Geometry check sheet. Reference: the model listing, model coordinates, mm. A direction names the side the tool comes from. Coordinates: 2 decimals unless noted, no trailing zeros. Write each loop counter-clockwise with the first axis right and the second up, starting at its lowest first coordinate (ties: lowest second). Pieces come first, ordered by that corner, then holes. Notation, with made-up numbers: (42, 42) -> (66, 42) arc R16 cw to (66, 55) -> close; hole circle Ø11 at (30.25, 85). An arc over 180 degrees is marked (long way). Answer in a Markdown table with one row per item. Add a question column.
1. Cross-section at B-B on x = 44.25. Record the cut outline in (y, z), and give its area (3 significant figures).
2. Mould release check, pull along Y, two halves, no side actions. Record for faces 1 (the flat face through (49, 18, 40.5)), 2 (the flat face through (-16, 2, -1)), 3 (the cylindrical face through (67.614, 28.25, 41.486)): pulls with the +Y half, pulls with the -Y half, needs draft (parallel to the pull), parting line crosses it, or undercut.
3. Depth check by flat-ended pin: P1, Ø17, axis at x = 40.5, y = 24, coming from the +Z side; P2, Ø1.5, axis at x = 50.5, y = 22.5, coming from the -Z side; P3, Ø3.5, axis at x = 33.25, y = 9, coming from the -Z side; P4, Ø2, axis at y = 1.5, z = 57.5, coming from the +X side. Enter the tip coordinate at first touch or a pass-through.
4. Cross-section at D-D on x = 9.25. Record the cut outline in (y, z).
5. Cross-section at A-A on z = -50. Record the cut outline in (x, y), and give its area (3 significant figures).
6. Cross-section at C-C on y = 4.5. Record the cut outline in (x, z), and give its area (3 significant figures).
7. Set-up check for faces 4 (the flat face through (48, 17, 42.5)), 5 (the cylindrical face through (67.614, 28.25, -41.514)): record each of +Z, -Z, +X, -X, +Y, -Y from which the full face is reachable in a straight line by a thin tool's end or side.
8. Scan lines: L1, parallel to Y at x = 66.25, z = 41.25; L2, parallel to X at y = 0.95, z = 71; L3, parallel to X at y = 1.6, z = -50. Record each from-to range of solid material in increasing order. Write a range as from..to.
```python
from build123d import *

# Parameters (mm, degrees)
SKETCH1_R           = 2.15
SKETCH1_R_2         = 1.75
SKETCH1_W           = 10.5
SKETCH1_H           = 6
SKETCH1_W_2         = 6
SKETCH1_H_2         = 4
SKETCH1_H_3         = 10.5
BOSS_EXTRUDE1_DEPTH = 2
SKETCH2_W           = 40
SKETCH2_H           = 2
BOSS_EXTRUDE2_DEPTH = 34
SKETCH4_R           = 1.85
SKETCH4_R_2         = 7.5
CUT_EXTRUDE2_DEPTH  = 120
SKETCH5_W           = 4.5
SKETCH5_H           = 32.5
CUT_EXTRUDE3_DEPTH  = 120


with BuildPart() as part:
    # Sketch1 → Boss-Extrude1 (new body)
    with BuildSketch(Plane(origin=(0, 0, 0), x_dir=(1, 0, 0), z_dir=(0, 1, 0))):
        Polygon((-68.75, -75), (33.25, -75), (33.25, -42.5), (68.75, -42.5), (68.75, 42.5), (33.25, 42.5), (33.25, 75), (-68.75, 75), align=None)
        with Locations(Location((-56.75, -71, 0), (0, 0, 270))):
            Circle(SKETCH1_R, mode=Mode.SUBTRACT)
        with Locations(Location((-41.97, -71, 0), (0, 0, 270))):
            Circle(SKETCH1_R, mode=Mode.SUBTRACT)
        with Locations(Location((-52.25, -40.5, 0), (0, 0, 270))):
            Circle(SKETCH1_R_2, mode=Mode.SUBTRACT)
        with Locations(Location((-29.75, -50, 0), (0, 0, 270))):
            Circle(SKETCH1_R_2, mode=Mode.SUBTRACT)
        with Locations(Location((-35.75, -19.5, 0), (0, 0, 270))):
            Circle(SKETCH1_R_2, mode=Mode.SUBTRACT)
        with Locations(Location((-26.5, -28.4, 0), (0, 0, 270))):
            Circle(SKETCH1_R_2, mode=Mode.SUBTRACT)
        with Locations(Location((-14.75, -37, 0), (0, 0, 270))):
            Circle(SKETCH1_R_2, mode=Mode.SUBTRACT)
        with Locations(Location((9.25, -50, 0), (0, 0, 270))):
            Circle(SKETCH1_R_2, mode=Mode.SUBTRACT)
        with Locations(Location((13.5, -68.4, 0), (0, 0, 270))):
            Circle(SKETCH1_R_2, mode=Mode.SUBTRACT)
        with Locations(Location((-52.25, 40.5, 0), (0, 0, 270))):
            Circle(SKETCH1_R_2, mode=Mode.SUBTRACT)
        with Locations(Location((-35.75, 19.5, 0), (0, 0, 270))):
            Circle(SKETCH1_R_2, mode=Mode.SUBTRACT)
        with Locations(Location((-56.75, 71, 0), (0, 0, 270))):
            Circle(SKETCH1_R, mode=Mode.SUBTRACT)
        with Locations(Location((-41.97, 71, 0), (0, 0, 270))):
            Circle(SKETCH1_R, mode=Mode.SUBTRACT)
        with Locations(Location((-29.75, 50, 0), (0, 0, 270))):
            Circle(SKETCH1_R_2, mode=Mode.SUBTRACT)
        with Locations(Location((-26.5, 28.4, 0), (0, 0, 270))):
            Circle(SKETCH1_R_2, mode=Mode.SUBTRACT)
        with Locations(Location((9.25, 50, 0), (0, 0, 270))):
            Circle(SKETCH1_R_2, mode=Mode.SUBTRACT)
        with Locations(Location((13.5, 68.4, 0), (0, 0, 270))):
            Circle(SKETCH1_R_2, mode=Mode.SUBTRACT)
        with Locations((-52, -61.25)):
            Rectangle(SKETCH1_W, SKETCH1_H, mode=Mode.SUBTRACT)
        with Locations((-49.92, -70)):
            Rectangle(SKETCH1_W_2, SKETCH1_H_2, mode=Mode.SUBTRACT)
        with Locations((-52, 61.25)):
            Rectangle(SKETCH1_W, SKETCH1_H, mode=Mode.SUBTRACT)
        with Locations((-49.92, 70)):
            Rectangle(SKETCH1_W_2, SKETCH1_H_2, mode=Mode.SUBTRACT)
        with Locations((61.796244223, 0)):
            Rectangle(SKETCH1_W_2, SKETCH1_H_3, mode=Mode.SUBTRACT)
    extrude(amount=BOSS_EXTRUDE1_DEPTH)

    # Sketch2 → Boss-Extrude2 (add)
    with BuildSketch(Plane(origin=(0, 0, 0), x_dir=(-1, 0, 0), z_dir=(0, -1, 0))):
        with Locations((-48.75, 41.5)):
            Rectangle(SKETCH2_W, SKETCH2_H)
        with Locations((-48.75, -41.5)):
            Rectangle(SKETCH2_W, SKETCH2_H)
    extrude(amount=-BOSS_EXTRUDE2_DEPTH)

    # Sketch4 → Cut-Extrude2 (cut)
    with BuildSketch(Plane(origin=(0, 0, -42.5), x_dir=(-1, 0, 0), z_dir=(0, 0, -1))):
        with Locations((-66.25, 27)):
            Circle(SKETCH4_R)
        with Locations((-33.25, 27)):
            Circle(SKETCH4_R)
        with Locations((-33.25, 9)):
            Circle(SKETCH4_R)
        with Locations((-66.25, 9)):
            Circle(SKETCH4_R)
        with Locations((-57.25, 18)):
            Circle(SKETCH4_R_2)
        with BuildLine():
            Line((-47, 13), (-47, 23))
            ThreePointArc((-47, 23), (-44.25, 25.75), (-41.5, 23))
            Line((-41.5, 23), (-41.5, 13))
            ThreePointArc((-41.5, 13), (-44.25, 10.25), (-47, 13))
        make_face()
    extrude(amount=-CUT_EXTRUDE2_DEPTH, mode=Mode.SUBTRACT)

    # Sketch5 → Cut-Extrude3 (cut)
    with BuildSketch(Plane(origin=(0, 2, 0), x_dir=(1, 0, 0), z_dir=(0, 1, 0))):
        with Locations((31, -58.75)):
            Rectangle(SKETCH5_W, SKETCH5_H)
        with Locations((31, 58.75)):
            Rectangle(SKETCH5_W, SKETCH5_H)
    extrude(amount=-CUT_EXTRUDE3_DEPTH, mode=Mode.SUBTRACT)


solid = part.part
```
Results found:
| question | item | result |
|---|---|---|
| 1 | outline | (0, -42.5) -> (10.25, -42.5) -> (10.25, -40.5) -> (2, -40.5) -> (2, 40.5) -> (10.25, 40.5) -> (10.25, 42.5) -> (0, 42.5) -> close; (25.75, -42.5) -> (34, -42.5) -> (34, -40.5) -> (25.75, -40.5) -> close; (25.75, 40.5) -> (34, 40.5) -> (34, 42.5) -> (25.75, 42.5) -> close |
| 1 | area | 236 mm^2 |
| 2 | face 1 | needs draft |
| 2 | face 2 | pulls with the +Y half |
| 2 | face 3 | undercut |
| 3 | P1 | stops at z = 42.5 |
| 3 | P2 | stops at z = -42.5 |
| 3 | P3 | passes through |
| 3 | P4 | stops at x = 28.75 |
| 4 | outline | (0, -75) -> (2, -75) -> (2, -51.75) -> (0, -51.75) -> close; (0, -48.25) -> (2, -48.25) -> (2, 48.25) -> (0, 48.25) -> close; (0, 51.75) -> (2, 51.75) -> (2, 75) -> (0, 75) -> close |
| 5 | outline | (-68.75, 0) -> (-31.5, 0) -> (-31.5, 2) -> (-68.75, 2) -> close; (-28, 0) -> (7.5, 0) -> (7.5, 2) -> (-28, 2) -> close; (11, 0) -> (28.75, 0) -> (28.75, 2) -> (11, 2) -> close |
| 5 | area | 181 mm^2 |
| 6 | outline | (28.75, -42.5) -> (68.75, -42.5) -> (68.75, -40.5) -> (28.75, -40.5) -> close; (28.75, 40.5) -> (68.75, 40.5) -> (68.75, 42.5) -> (28.75, 42.5) -> close |
| 6 | area | 160 mm^2 |
| 7 | face 4 | +Z, +X, +Y, -Y |
| 7 | face 5 | +Z, -Z |
| 8 | L1 | y = 0..7.15, 10.85..25.15, 28.85..34 |
| 8 | L2 | x = -68.75..-58.9, -54.6..-52.92, -46.92..-44.12, -39.82..28.75 |
| 8 | L3 | x = -68.75..-31.5, -28..7.5, 11..28.75 |
